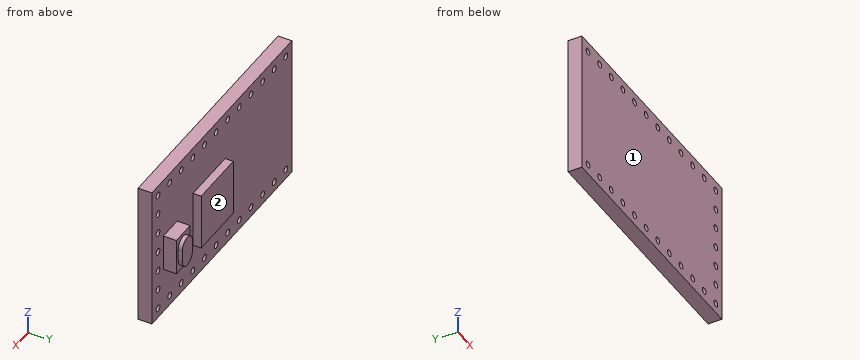
```python
from build123d import *

# Parameters (mm, degrees)
ESQUISSE1_W             = 30.6
ESQUISSE1_H             = 17.7
BOSS_EXTRU_1_DEPTH      = 1.7
ESQUISSE2_W             = 7
ESQUISSE2_H             = 7
BOSS_EXTRU_2_DEPTH      = 1
ESQUISSE3_R             = 0.4
ENL_V_MAT_EXTRU_1_DEPTH = 3.7
ESQUISSE4_W             = 3
ESQUISSE4_H             = 4.5
BOSS_EXTRU_3_DEPTH      = 1.6
BOSS_EXTRU_4_DEPTH      = 0.5


with BuildPart() as part:
    # Esquisse1 → Boss.-Extru.1 (new body)
    with BuildSketch(Plane(origin=(0, 0, 0), x_dir=(1, 0, 0), z_dir=(0, 1, 0))):
        Rectangle(ESQUISSE1_W, ESQUISSE1_H)
    extrude(amount=BOSS_EXTRU_1_DEPTH)

    # Esquisse2 → Boss.-Extru.2 (add)
    with BuildSketch(Plane(origin=(0, 1.7, 0), x_dir=(1, 0, 0), z_dir=(0, 1, 0))):
        with Locations((2.8, 0.75)):
            Rectangle(ESQUISSE2_W, ESQUISSE2_H)
    extrude(amount=BOSS_EXTRU_2_DEPTH)

    # Esquisse3 → Enlèv. mat.-Extru.1 (cut, through all)
    with BuildSketch(Plane.XZ):
        with Locations((-13.97, -7.62)):
            Circle(ESQUISSE3_R)
        with Locations((-11.43, -7.62)):
            Circle(ESQUISSE3_R)
        with Locations((-8.89, -7.62)):
            Circle(ESQUISSE3_R)
        with Locations((-6.35, -7.62)):
            Circle(ESQUISSE3_R)
        with Locations((-3.81, -7.62)):
            Circle(ESQUISSE3_R)
        with Locations((-1.27, -7.62)):
            Circle(ESQUISSE3_R)
        with Locations((1.27, -7.62)):
            Circle(ESQUISSE3_R)
        with Locations((3.81, -7.62)):
            Circle(ESQUISSE3_R)
        with Locations((6.35, -7.62)):
            Circle(ESQUISSE3_R)
        with Locations((8.89, -7.62)):
            Circle(ESQUISSE3_R)
        with Locations((11.43, -7.62)):
            Circle(ESQUISSE3_R)
        with Locations((13.97, -7.62)):
            Circle(ESQUISSE3_R)
        with Locations((13.97, -5.08)):
            Circle(ESQUISSE3_R)
        with Locations((13.97, -2.54)):
            Circle(ESQUISSE3_R)
        with Locations((13.97, 0)):
            Circle(ESQUISSE3_R)
        with Locations((13.97, 2.54)):
            Circle(ESQUISSE3_R)
        with Locations((13.97, 5.08)):
            Circle(ESQUISSE3_R)
        with Locations((13.97, 7.62)):
            Circle(ESQUISSE3_R)
        with Locations((11.43, 7.62)):
            Circle(ESQUISSE3_R)
        with Locations((8.89, 7.62)):
            Circle(ESQUISSE3_R)
        with Locations((6.35, 7.62)):
            Circle(ESQUISSE3_R)
        with Locations((3.81, 7.62)):
            Circle(ESQUISSE3_R)
        with Locations((1.27, 7.62)):
            Circle(ESQUISSE3_R)
        with Locations((-1.27, 7.62)):
            Circle(ESQUISSE3_R)
        with Locations((-3.81, 7.62)):
            Circle(ESQUISSE3_R)
        with Locations((-6.35, 7.62)):
            Circle(ESQUISSE3_R)
        with Locations((-8.89, 7.62)):
            Circle(ESQUISSE3_R)
        with Locations((-11.43, 7.62)):
            Circle(ESQUISSE3_R)
        with Locations((-13.97, 7.62)):
            Circle(ESQUISSE3_R)
    extrude(amount=-ENL_V_MAT_EXTRU_1_DEPTH, mode=Mode.SUBTRACT)

    # Esquisse4 → Boss.-Extru.3 (add)
    with BuildSketch(Plane(origin=(0, 1.7, 0), x_dir=(1, 0, 0), z_dir=(0, 1, 0))):
        with Locations((11.3, 0.9)):
            Rectangle(ESQUISSE4_W, ESQUISSE4_H)
    extrude(amount=BOSS_EXTRU_3_DEPTH)

    # Esquisse5 → Boss.-Extru.4 (add)
    with BuildSketch(Plane(origin=(0, 3.3, 0), x_dir=(1, 0, 0), z_dir=(0, 1, 0))):
        with BuildLine():
            Line((12.4, 1.65), (12.4, 0.15))
            ThreePointArc((12.4, 0.15), (11.3, -0.95), (10.2, 0.15))
            Line((10.2, 0.15), (10.2, 1.65))
            ThreePointArc((10.2, 1.65), (11.3, 2.75), (12.4, 1.65))
        make_face()
    extrude(amount=BOSS_EXTRU_4_DEPTH)


solid = part.part
```
Here's how the part is built. I have some questions about the finished solid (model axes, mm). Face numbers are marked on the shaded views. A direction names the side the tool comes from. Coordinates: 2 decimals unless noted, no trailing zeros. Loops run counter-clockwise (first coordinate to the right, second up) from the corner with the lowest first, then second, coordinate; pieces in that order, holes last. Notation, with made-up numbers: (85.25, 4) -> (132.25, 4) arc R25 ccw to (132.25, 36) -> close; hole circle Ø9 at (31.5, -4.5). An arc over 180 degrees is marked (long way). Return JSON: item names as keys, results as strings.
1) If we section it at A-A, the plane y = 2: Write out the boundary of the cut face in (x, z), then the cut area to 3 significant figures.
Results below:
{"outline": "(-0.7, -4.25) -> (6.3, -4.25) -> (6.3, 2.75) -> (-0.7, 2.75) -> close; (9.8, -3.15) -> (12.8, -3.15) -> (12.8, 1.35) -> (9.8, 1.35) -> close", "area": "62.5 mm²"}
2) If we section it at B-B, the plane z = 5.08: Write out the boundary of the cut face in (x, y), then the cut area to 3 significant figures.
Results below:
{"outline": "(-15.3, 0) -> (13.57, 0) -> (13.57, 1.7) -> (-15.3, 1.7) -> close; (14.37, 0) -> (15.3, 0) -> (15.3, 1.7) -> (14.37, 1.7) -> close", "area": "50.7 mm²"}
3) Will these pins go through, and if not, where does the flat tip stop? pin 1 (2 mm diameter, centred on x = -9, z = -6.5, fed in from +Y); pin 2 (3.5 mm diameter, centred on x = 3.5, z = -1, fed in from +Y); pin 3 (0.8 mm diameter, centred on x = 11, y = 2.5, fed in from -Z).
Results below:
{"pin 1": "y = 1.7", "pin 2": "y = 2.7", "pin 3": "z = -3.15"}
4) If we section it at C-C, the plane x = 13.97: Count the separate pieces of the cut face and the enclosed holes in it, then the cut area to 3 significant figures.
Results below:
{"separate pieces": "8", "enclosed holes": "0", "area": "20.6 mm²"}
5) I need wall thicknesses on line 1 (Z direction, x = -13.97, y = 0.8); line 2 (X direction, y = 1.75, z = 0); line 3 (Y direction, x = -3, z = -7.5). Which ranges of each line are inside material? Lowest first, please. Write a range as from..to.
Results below:
{"line 1": "-8.85..-8.02, -7.22..7.22, 8.02..8.85", "line 2": "-0.7..6.3, 9.8..12.8", "line 3": "0..1.7"}
6) For the marked faces 1 and 2, which set-ups out of +Z, -Z, +X, -X, +Y, -Y let a thin tool reach every point of the face, with its end or its side?
Results below:
{"face 1": "+Z, -Z, +X, -X, -Y", "face 2": "+Z, -Z, -X, +Y"}
